Part model, mm, in its own coordinate system. A direction names the side the tool comes from. Round coordinates to 2 decimals unless told otherwise and drop trailing zeros. Order: outer loops, then holes, each group sorted by start corner. A loop starts at its lowest first (then second) coordinate and runs counter-clockwise, first axis right, second up. Notation, with made-up numbers: (-25, -23) - (10, -23) arc R13 cw to (10, -8) - close; hole circle Ø8 at (4, 14.25). An arc over 180 degrees is marked (long way). Answer as a JSON object with one key per item and string values.
```python
from build123d import *

# Parameters (mm, degrees)
SKETCH004_R           = 54
EXTRUDE004_DEPTH      = 20
SKETCH003_R           = 10
EXTRUDE003_DEPTH      = 30
EXTRUDE003_DEPTH_BACK = 14
SKETCH005_R           = 7
EXTRUDE005_DEPTH      = 20


with BuildPart() as outercylinder:
    # Sketch004 (on Face3 of Extrude003) → Extrude004 (new body)
    with BuildSketch(Plane.XY.offset(98.4)):
        with Locations((-58.7, 20.37)):
            Circle(SKETCH004_R)
    extrude(amount=-EXTRUDE004_DEPTH)


with BuildPart() as innercylinder:
    # Sketch003 (on Face4 of Extrude002) → Extrude003 (new body, two sides)
    with BuildSketch(Plane.XY.offset(68.4)) as extrude003_sk:
        with Locations((-58.7, 20.37)):
            Circle(SKETCH003_R)
    extrude(amount=EXTRUDE003_DEPTH)
    extrude(extrude003_sk.sketch, amount=-EXTRUDE003_DEPTH_BACK)


with BuildPart() as motoradapter:
    # Sketch005 (on Face3 of Extrude003) → Extrude005 (new body)
    with BuildSketch(Plane.XY.offset(98.4)):
        with Locations((-58.7, 20.37)):
            Circle(SKETCH005_R)
    extrude(amount=EXTRUDE005_DEPTH)

    # Fusion005: union outerCylinder, innerCylinder
    add(outercylinder.part)
    add(innercylinder.part)


solid = motoradapter.part
```
Item 1: Cut at B-B (x = -58.7). Write the cut outline in (y, z), plus the area to 3 significant figures.
Taken from the geometry:
{"outline": "(-33.63, 78.4) - (10.37, 78.4) - (10.37, 54.4) - (30.37, 54.4) - (30.37, 78.4) - (74.37, 78.4) - (74.37, 98.4) - (27.37, 98.4) - (27.37, 118.4) - (13.37, 118.4) - (13.37, 98.4) - (-33.63, 98.4) - close", "area": "2,920 mm2"}
Item 2: Cut at D-D (z = 101.5). Write the cut outline in (x, y), plus the area to 3 significant figures.
Taken from the geometry:
{"outline": "circle Ø14 at (-58.7, 20.37)", "area": "154 mm2"}
Item 3: Tool access for faces 1 (the cylindrical face through (-66.07, 27.13, 66.57)), 2 (the flat face through (-59, 21, 54.4)), 3 (the cylindrical face through (-54.937, 26.272, 108.26)): list every direction of +Z, -Z, +X, -X, +Y, -Y with a clear straight run to the whole face (end or side of a thin tool).
Taken from the geometry:
{"face 1": "-Z", "face 2": "-Z, +X, -X, +Y, -Y", "face 3": "+Z"}
Item 4: Cut at C-C (z = 94). Write the cut outline in (x, y), plus the area to 3 significant figures.
Taken from the geometry:
{"outline": "circle Ø108 at (-58.7, 20.37)", "area": "9,160 mm2"}
Item 5: Cut at A-A (y = 20.37). Write the cut outline in (x, z), plus the area to 3 significant figures.
Taken from the geometry:
{"outline": "(-112.7, 78.4) - (-68.7, 78.4) - (-68.7, 54.4) - (-48.7, 54.4) - (-48.7, 78.4) - (-4.7, 78.4) - (-4.7, 98.4) - (-51.7, 98.4) - (-51.7, 118.4) - (-65.7, 118.4) - (-65.7, 98.4) - (-112.7, 98.4) - close", "area": "2,920 mm2"}
Item 6: Drop flat-ended pins along their axis: P1, Ø1.5, axis at y = 14.5, z = 88, coming from the +X side; P2, Ø10, axis at x = -87.5, y = 9.5, coming from the -Z side; P3, Ø1.5, axis at y = -22.5, z = 87, coming from the +X side. Give the stop position or say it passes through.
Taken from the geometry:
{"P1": "x = -4.94", "P2": "z = 78.4", "P3": "x = -24.91"}
Item 7: Probe L1, parallel to Z at x = -82, y = 58; L2, parallel to Y at x = -26, z = 95; L3, parallel to Z at x = -49.5, y = 17. List the from-to ranges inside material, lowest first. Write a range as from..to.
Taken from the geometry:
{"L1": "78.4..98.4", "L2": "-22.6..63.34", "L3": "54.4..98.4"}
